Part model, mm, in its own coordinate system. Coordinates: 2 decimals unless noted, no trailing zeros. Write each loop counter-clockwise with the first axis right and the second up, starting at its lowest first coordinate (ties: lowest second). Pieces come first, ordered by that corner, then holes. Notation, with made-up numbers: (22.5, 76.25) -> (79.5, 76.25) arc R27 cw to (79.5, 100.25) -> close; hole circle Ø10 at (85.5, 46). An arc over 180 degrees is marked (long way). Write item = value, one per line. Start each with the question number.
Q1. Probe line 1 (Y direction, x = -25, z = 1.9); line 2 (X direction, y = 12, z = 0.4); line 3 (Y direction, x = 0, z = 1.1). List the from-to ranges inside material, lowest first.
Q2. Pin check, flat tips, straight feed: P1, Ø17.5, axis at x = 25, y = 0, coming from the -Z side; P2, Ø1.5, axis at y = 16, z = 1.5, coming from the +X side; P3, Ø1.5, axis at y = 2.5, z = 2, coming from the +X side. Stop position of each tip, or through.
Q3. Band-saw the part on A-A, the plane x = 0. List the corners of the cut face in (y, z).
Q4. Band-saw the part on C-C, the plane z = 1. List the corners of the cut face in (x, y).
Q5. Band-saw the part on B-B, the plane y = 0. List the corners of the cut face in (x, z).
Q6. Band-saw the part on D-D, the plane y = 6. List the corners of the cut face in (x, z), plus the area to 3 significant figures.
from build123d import *

# Parameters (mm, degrees)
F0_R     = 11
F0_W     = 10.189878
F0_H     = 10
F1_DEPTH = 3


with BuildPart() as f1:
    # F0 (on Top) → F1 (new body)
    with BuildSketch(Plane.XY):
        with BuildLine():
            Line((5.094939, 11.96), (-5.094939, 11.96))
            ThreePointArc((-5.094939, 11.96), (-9.192388, 9.192388), (-11.96, 5.094939))
            ThreePointArc((-11.96, 5.094939), (-39, 0), (-11.96, -5.094939))
            ThreePointArc((-11.96, -5.094939), (-9.192388, -9.192388), (-5.094939, -11.96))
            Line((-5.094939, -11.96), (5.094939, -11.96))
            ThreePointArc((5.094939, -11.96), (9.192388, -9.192388), (11.96, -5.094939))
            ThreePointArc((11.96, -5.094939), (39, 0), (11.96, 5.094939))
            ThreePointArc((11.96, 5.094939), (9.192388, 9.192388), (5.094939, 11.96))
        make_face()
        with Locations((-25, 0)):
            Circle(F0_R, mode=Mode.SUBTRACT)
        Circle(F0_R, mode=Mode.SUBTRACT)
        with Locations((25, 0)):
            Circle(F0_R, mode=Mode.SUBTRACT)
        with Locations((0, 16.96)):
            Rectangle(F0_W, F0_H)
        with Locations((0, -16.96)):
            Rectangle(F0_W, F0_H)
    extrude(amount=F1_DEPTH)


solid = f1.part
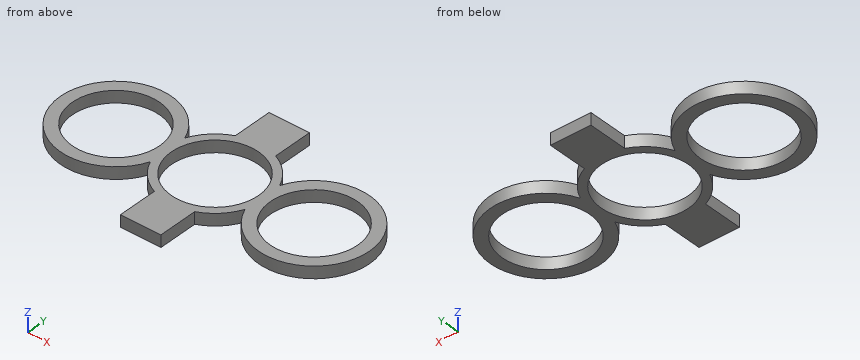
Ans:
q1.line_1 = -14 to -11, 11 to 14
q1.line_2 = -32.21 to -17.79, -5.09 to 5.09, 17.79 to 32.21
q1.line_3 = -21.96 to -11, 11 to 21.96
q2.P1 = through
q2.P2 = 5.09
q2.P3 = 38.89
q3.outline = (-21.96, 0) -> (-11, 0) -> (-11, 3) -> (-21.96, 3) -> close; (11, 0) -> (21.96, 0) -> (21.96, 3) -> (11, 3) -> close
q4.outline = (-11.96, -5.09) arc R13 ccw to (-5.09, -11.96) -> (-5.09, -21.96) -> (5.09, -21.96) -> (5.09, -11.96) arc R13 ccw to (11.96, -5.09) arc R14 ccw (long way) to (11.96, 5.09) arc R13 ccw to (5.09, 11.96) -> (5.09, 21.96) -> (-5.09, 21.96) -> (-5.09, 11.96) arc R13 ccw to (-11.96, 5.09) arc R14 ccw (long way) to start; hole circle Ø22 at (-25, 0); hole circle Ø22 at (0, 0); hole circle Ø22 at (25, 0)
q5.outline = (-39, 0) -> (-36, 0) -> (-36, 3) -> (-39, 3) -> close; (-14, 0) -> (-11, 0) -> (-11, 3) -> (-14, 3) -> close; (11, 0) -> (14, 0) -> (14, 3) -> (11, 3) -> close; (36, 0) -> (39, 0) -> (39, 3) -> (36, 3) -> close
q6.outline = (-37.65, 0) -> (-34.22, 0) -> (-34.22, 3) -> (-37.65, 3) -> close; (-15.78, 0) -> (-12.35, 0) -> (-12.35, 3) -> (-15.78, 3) -> close; (-11.53, 0) -> (-9.22, 0) -> (-9.22, 3) -> (-11.53, 3) -> close; (9.22, 0) -> (11.53, 0) -> (11.53, 3) -> (9.22, 3) -> close; (12.35, 0) -> (15.78, 0) -> (15.78, 3) -> (12.35, 3) -> close; (34.22, 0) -> (37.65, 0) -> (37.65, 3) -> (34.22, 3) -> close
q6.area = 55.0 mm2
